```python
from build123d import *

# Parameters (mm, degrees)
F0_W     = 114.3
F0_H     = 203.2
F1_DEPTH = 76.2
F2_T     = -2.54
F3_R     = 12.7


with BuildPart() as f1:
    # F0 (on Top) → F1 (new body)
    with BuildSketch(Plane.XY):
        with Locations((0, 38.1)):
            Rectangle(F0_W, F0_H)
    extrude(amount=F1_DEPTH)

    # F2
    f2_openings = [f1.faces().sort_by_distance(p)[0] for p in [
        (0, 38.1, 76.2),
    ]]
    offset(amount=F2_T, openings=f2_openings)

    # F3
    f3_edges = [f1.edges().sort_by_distance(p)[0] for p in [
        (-54.61, -60.96, 39.37),
    ]]
    fillet(f3_edges, radius=F3_R)


solid = f1.part
```
Source: CAD feature listing. Evaluate the final solid. Frame: model axes, mm. A direction names the side the tool comes from. Give positions to 0.01 mm unless a question says otherwise; leave off trailing zeros. Loops run counter-clockwise (first coordinate to the right, second up) from the corner with the lowest first, then second, coordinate; pieces in that order, holes last. Notation, with made-up numbers: (86.25, 21.5) -> (115.25, 21.5) arc R33 cw to (115.25, 49.5) -> close; hole circle Ø7 at (63, -2). An arc over 180 degrees is marked (long way). Use a Markdown table: item, result. Add a question column.
(1) Access query for faces 1 (the face through (-1, 39, 2.54)), 2 (the face through (-55, 39, 76.2)). Directions: +Z, -Z, +X, -X, +Y, -Y. A direction counts if a zero-diameter tool reaches every point of the face in a straight line with its end or side. Return the directions, or none.
(2) Section query B-B (y = 1). Output: boundary loops of the cut face in (x, z), then the cut area to 3 significant figures.
(3) First-contact query: pin 1 Ø2 at (x, y) = (19.5, 76.5) entering from +Z. Flat tip, straight axial feed; report the tip coordinate or a pass-through.
(4) Ray query, line 1 (X direction, y = -36, z = 66.5); line 2 (Y direction, x = -1, z = 17); line 3 (Z direction, x = 47.5, y = 35.5). Return the intervals inside material, ascending.
(5) Pull-direction query (Y, two-part tool) for faces 3 (the face through (-1, 139.7, 38)), 4 (the face through (-1, 137.16, 39)), 5 (the face through (-1, -63.5, 38)), 6 (the face through (-1, 40, 0)); classes: +Y half, -Y half, draft (parallel to the pull), parting line (faces both ways), or undercut.
(6) Section query C-C (x = 34). Output: boundary loops of the cut face in (y, z).
(7) Section query A-A (z = 22.5). Output: boundary loops of the cut face in (x, y), then the cut area to 3 significant figures.
Checked values:
| question | item | result |
|---|---|---|
| 1 | face 1 | +Z |
| 1 | face 2 | +Z, +X, -X, +Y, -Y |
| 2 | outline | (-57.15, 0) -> (57.15, 0) -> (57.15, 76.2) -> (54.61, 76.2) -> (54.61, 2.54) -> (-54.61, 2.54) -> (-54.61, 76.2) -> (-57.15, 76.2) -> close |
| 2 | area | 665 mm^2 |
| 3 | pin 1 | z = 2.54 |
| 4 | line 1 | -57.15 to -54.61, 54.61 to 57.15 |
| 4 | line 2 | -63.5 to -60.96, 137.16 to 139.7 |
| 4 | line 3 | 0 to 2.54 |
| 5 | face 3 | +Y half |
| 5 | face 4 | undercut |
| 5 | face 5 | -Y half |
| 5 | face 6 | draft |
| 6 | outline | (-63.5, 0) -> (139.7, 0) -> (139.7, 76.2) -> (137.16, 76.2) -> (137.16, 2.54) -> (-60.96, 2.54) -> (-60.96, 76.2) -> (-63.5, 76.2) -> close |
| 7 | outline | (-57.15, -63.5) -> (57.15, -63.5) -> (57.15, 139.7) -> (-57.15, 139.7) -> close; hole (-54.61, -48.26) arc R12.7 ccw to (-41.91, -60.96) -> (54.61, -60.96) -> (54.61, 137.16) -> (-54.61, 137.16) -> close |
| 7 | area | 1,620 mm^2 |
